```python
from build123d import *

# Parameters (mm, degrees)
F1_DEPTH = 20
F3_D     = 12
F3_DEPTH = 25
F3_TIP   = 3.6051637142


with BuildPart() as f1:
    # F0 (on Top) → F1 (new body)
    with BuildSketch(Plane.XY):
        with BuildLine():
            ThreePointArc((0, -7.5), (-7.5, 0), (0, 7.5))
            Line((0, 7.5), (-44.8082763299, 7.5))
            Line((-44.8082763299, 7.5), (-44.8082763299, -7.5))
            Line((-44.8082763299, -7.5), (0, -7.5))
        make_face()
    extrude(amount=F1_DEPTH)

    # F3
    with Locations(Plane(origin=(-44.8082763299, 0, 0), x_dir=(0, -1, 0), z_dir=(-1, 0, 0))):
        with Locations((0, 10)):
            Hole(F3_D / 2, depth=F3_DEPTH)
            with Locations((0, 0, -(F3_DEPTH + F3_TIP / 2))):  # 118° drill point
                Cone(0, F3_D / 2, F3_TIP, mode=Mode.SUBTRACT)


solid = f1.part
```
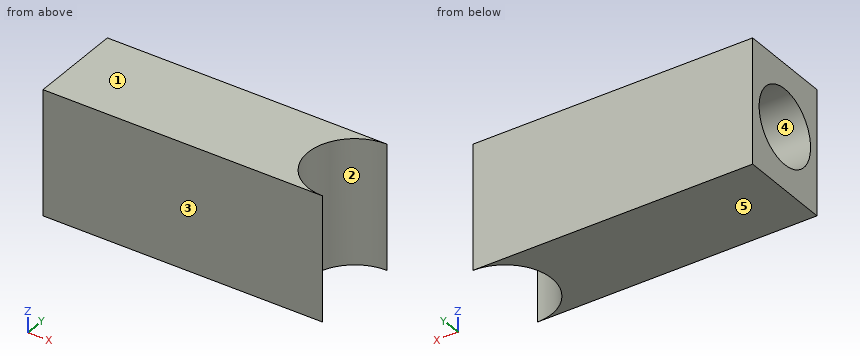
Read the model definition and answer for the solid it produces. Units are mm, in the model's axes. Face numbers are marked on the shaded views. A direction names the side the tool comes from. Coordinates: 2 decimals unless noted, no trailing zeros. Order: outer loops, then holes, each group sorted by start corner. A loop starts at its lowest first (then second) coordinate and runs counter-clockwise, first axis right, second up. Notation, with made-up numbers: (77.25, -5.75) - (119.25, -5.75) arc R22 ccw to (119.25, 31.25) - close; hole circle Ø8 at (89, 69). An arc over 180 degrees is marked (long way). Answer as a JSON object with one key per item and string values. Group by question number.
Item 1: Section B-B (z = 18.5) is taken. Give the vertices of the cut face in (x, y), plus the area to 3 significant figures.
Item 2: Flat-ended cylindrical pins translate along their axes: P1, Ø3, axis at x = -5.5, y = -2, coming from the -Z side; P2, Ø2, axis at y = -5.5, z = 6, coming from the +X side; P3, Ø2, axis at y = 3.5, z = 4, coming from the +X side. Find the tip coordinate at first contact, or state that the pin passes through.
Item 3: The mould has two halves that part along Y. Classify the marked faces 1, 2 and 3: +Y half, -Y half, draft (parallel to the pull), parting line (faces both ways), or undercut.
Item 4: Section A-A (x = -27.5) is taken. Give the vertices of the cut face in (y, z).
Item 5: A tool of negligible diameter and unlimited length cuts with its end or side. For the marked faces 4 and 5, from which of +Z, -Z, +X, -X, +Y, -Y can it reach the whole face along a straight path? Write none if from no direction.
Item 6: Consider probe 1 along Y at (x, z) = (-26.75, 10); probe 2 along Z at (x, y) = (-39.5, 0); probe 3 along Y at (x, z) = (-40.5, 15.5). Determine where each line is inside the solid, lowest interval first. Write a range as from..to.
Item 7: Section C-C (x = -18.5) is taken. Give the vertices of the cut face in (y, z).
Results are:
{
 "1": {"outline": "(-44.81, -7.5) - (0, -7.5) arc R7.5 cw to (0, 7.5) - (-44.81, 7.5) - close", "area": "584 mm^2"},
 "2": {"P1": "passes through", "P2": "stops at x = -3.74", "P3": "stops at x = -6"},
 "3": {"face 1": "draft", "face 2": "undercut", "face 3": "-Y half"},
 "4": {"outline": "(-7.5, 0) - (7.5, 0) - (7.5, 20) - (-7.5, 20) - close; hole circle Ø12 at (0, 10)"},
 "5": {"face 4": "-X", "face 5": "-Z, +X, -X, +Y, -Y"},
 "6": {"probe 1": "y = -7.5..-6, 6..7.5", "probe 2": "z = 0..4, 16..20", "probe 3": "y = -7.5..-2.4, 2.4..7.5"},
 "7": {"outline": "(-7.5, 0) - (7.5, 0) - (7.5, 20) - (-7.5, 20) - close; hole circle Ø7.65 at (0, 10)"}
}
